```python
from build123d import *

# Parameters (mm, degrees)
F0_W     = 60.25
F0_H     = 40
F1_DEPTH = 1.7
F2_R     = 1.524
F3_DEPTH = 1.701
F4_W     = 14.732
F4_H     = 14.732
F5_DEPTH = 12.7


with BuildPart() as f1:
    # F0 (on Top) → F1 (new body)
    with BuildSketch(Plane.XY):
        Rectangle(F0_W, F0_H)
    extrude(amount=F1_DEPTH)

    # F2 (on face) → F3 (cut, through all)
    with BuildSketch(Plane.XY.offset(1.7)):
        with Locations((-28, 17.875)):
            Circle(F2_R)
        with Locations((28, 17.875)):
            Circle(F2_R)
        with Locations((28, -17.875)):
            Circle(F2_R)
        with Locations((-28, -17.875)):
            Circle(F2_R)
    extrude(amount=-F3_DEPTH, mode=Mode.SUBTRACT)

    # F4 (on face) → F5 (join)
    with BuildSketch(Plane.XY.offset(1.7)):
        with Locations((-22.759, 1.6)):
            Rectangle(F4_W, F4_H)
    extrude(amount=F5_DEPTH)


solid = f1.part
```
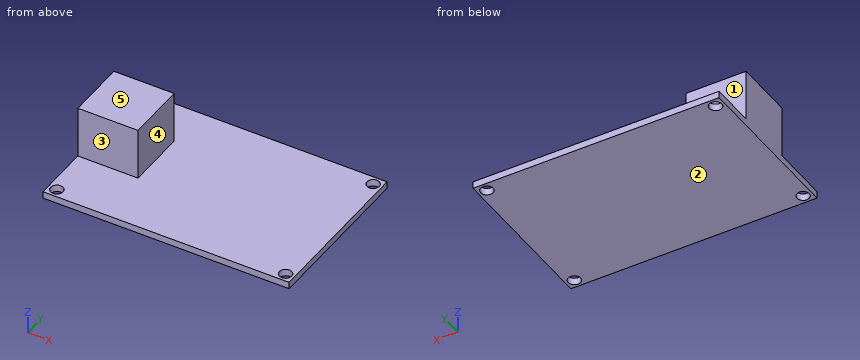
Part model, mm, in its own coordinate system. Face numbers are marked on the shaded views. A direction names the side the tool comes from. Give positions to 0.01 mm unless a question says otherwise; leave off trailing zeros. Loops run counter-clockwise (first coordinate to the right, second up) from the corner with the lowest first, then second, coordinate; pieces in that order, holes last. Notation, with made-up numbers: M -5,-16 L 19,-16 A19 cw 19,-4 Z; hole C 14,46 d5. An arc over 180 degrees is marked long. Return JSON: item names as keys, results as strings.
1) Flat gauge pins, fed straight in: pin 1 Ø5 at (x, z) = (-2.5, 4) entering from -Y; pin 2 Ø5 at (y, z) = (-6.5, 6) entering from +X; pin 3 Ø4 at (x, y) = (28, -17.875) entering from +Z. Where does each tip first touch, or does it go through?
Calculated:
{"pin 1": "stops at y = -20", "pin 2": "stops at x = -15.39", "pin 3": "stops at z = 1.7"}
2) Saw through at A-A, the plane x = -28. List the corners of the cut face in (y, z).
Calculated:
{"outline": "M -20,0 L -19.4,0 L -19.4,1.7 L -20,1.7 Z; M -16.35,0 L 16.35,0 L 16.35,1.7 L 8.97,1.7 L 8.97,14.4 L -5.77,14.4 L -5.77,1.7 L -16.35,1.7 Z; M 19.4,0 L 20,0 L 20,1.7 L 19.4,1.7 Z"}
3) 3-axis set-ups, long thin cutter, end or side, ignore diameter. For the marked faces 1, 2, 3, 4 and 5: which of +Z, -Z, +X, -X, +Y, -Y reach the whole face in a straight line?
Calculated:
{"face 1": "+Z, +X, -X, +Y", "face 2": "-Z, +X, -X, +Y, -Y", "face 3": "+Z, +X, -X, -Y", "face 4": "+Z, +X, +Y, -Y", "face 5": "+Z, +X, -X, +Y, -Y"}
4) Saw through at C-C, the plane y = 7. List the corners of the cut face in (x, z) (3 decimals), then the cut area to 3 significant figures.
Calculated:
{"outline": "M -30.125,0 L 30.125,0 L 30.125,1.7 L -15.393,1.7 L -15.393,14.4 L -30.125,14.4 Z", "area": "290 mm2"}
5) Saw through at D-D, the plane x = -20. List the corners of the cut face in (y, z), then the cut area to 3 significant figures.
Calculated:
{"outline": "M -20,0 L 20,0 L 20,1.7 L 8.97,1.7 L 8.97,14.4 L -5.77,14.4 L -5.77,1.7 L -20,1.7 Z", "area": "255 mm2"}
6) Drill centre lines: line 1 (Y direction, x = 28, z = 0.45); line 2 (Z direction, x = 17.5, y = -11.5); line 3 (X direction, y = 3.5, z = 11) (3 decimals). Where is each one in solid material? Low to high.
Calculated:
{"line 1": "y = -20 to -19.4, -16.35 to 16.35, 19.4 to 20", "line 2": "z = 0 to 1.7", "line 3": "x = -30.125 to -15.393"}
7) Saw through at B-B, the plane x = 28. List the corners of the cut face in (y, z).
Calculated:
{"outline": "M -20,0 L -19.4,0 L -19.4,1.7 L -20,1.7 Z; M -16.35,0 L 16.35,0 L 16.35,1.7 L -16.35,1.7 Z; M 19.4,0 L 20,0 L 20,1.7 L 19.4,1.7 Z"}
